The listing builds one solid part. Answer for the finished solid, in the listing's coordinates (mm). Face numbers are marked on the shaded views. A direction names the side the tool comes from. Coordinates: 2 decimals unless noted, no trailing zeros. Loops run counter-clockwise (first coordinate to the right, second up) from the corner with the lowest first, then second, coordinate; pieces in that order, holes last. Notation, with made-up numbers: (23.25, 70) -> (30.25, 70) arc R28 cw to (30.25, 88) -> close; hole circle Ø1 at (0.25, -17). An arc over 180 degrees is marked (long way). Answer in a Markdown table with one row per item.
```python
from build123d import *

# Parameters (mm, degrees)
F0_R       = 22.225
F1_DEPTH   = 76.2
F0_R_2     = 31.75
F2_DEPTH   = 50
F3_SIZE    = 3
F9_D       = 6.8
F9_ON_F7_D = 6.8


with BuildPart() as f1:
    # F0 (on Top) → F1 (new body)
    with BuildSketch(Plane.XY):
        Circle(F0_R)
    extrude(amount=-F1_DEPTH)

    # F0 (on Top) → F2 (join)
    with BuildSketch(Plane.XY):
        Circle(F0_R_2)
        Circle(F0_R, mode=Mode.SUBTRACT)
        Circle(F0_R)
    extrude(amount=F2_DEPTH)

    # F3
    f3_edges = [f1.edges().sort_by_distance(p)[0] for p in [
        (-31.75, 0, 50),
        (-22.225, 0, -76.2),
    ]]
    chamfer(f3_edges, length=F3_SIZE)

    # F9 (through all)
    with Locations(Plane.XZ.offset(31.75)):
        with Locations((0, 25)):
            Hole(F9_D / 2)

    # F9 on F7 (through all)
    with Locations(Plane.YZ.offset(31.75)):
        with Locations((0, 25)):
            Hole(F9_ON_F7_D / 2)


solid = f1.part
```
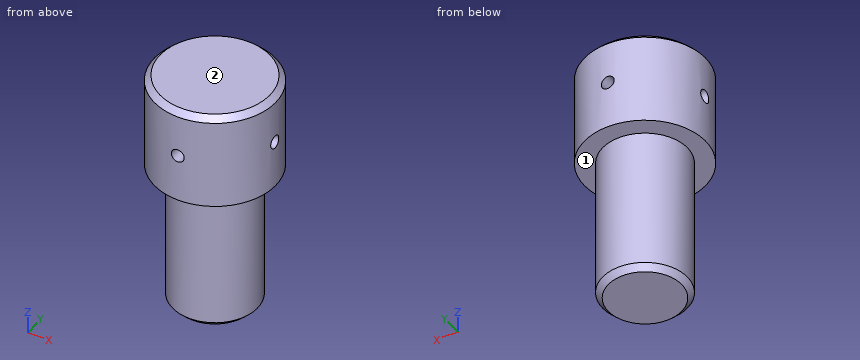
Item 1: A tool of negligible diameter and unlimited length cuts with its end or side. For the marked faces 1 and 2, from which of +Z, -Z, +X, -X, +Y, -Y can it reach the whole face along a straight path? Write none if from no direction.
Findings below:
| item | result |
|---|---|
| face 1 | -Z |
| face 2 | +Z, +X, -X, +Y, -Y |
Item 2: A cutting plane is placed at A-A, the plane z = 25. Determine the outline of the cut face in (x, y).
Findings below:
| item | result |
|---|---|
| outline | (-31.57, -3.4) arc R31.75 ccw to (-3.4, -31.57) -> (-3.4, -3.4) -> close; (-31.57, 3.4) -> (-3.4, 3.4) -> (-3.4, 31.57) arc R31.75 ccw to start; (3.4, -31.57) arc R31.75 ccw to (31.57, -3.4) -> (3.4, -3.4) -> close; (3.4, 3.4) -> (31.57, 3.4) arc R31.75 ccw to (3.4, 31.57) -> close |
Item 3: Find the intervals of material crossed by probe 1 along Z at (x, y) = (-13, 0); probe 2 along Z at (x, y) = (-11, 21); probe 3 along Y at (x, z) = (15.5, 25), in increasing order.
Findings below:
| item | result |
|---|---|
| probe 1 | z = -76.2 to 21.6, 28.4 to 50 |
| probe 2 | z = 0 to 50 |
| probe 3 | y = -27.71 to -3.4, 3.4 to 27.71 |
Item 4: Flat-ended cylindrical pins translate along their axes: pin 1 Ø10 at (x, z) = (8.5, -15) entering from +Y; pin 2 Ø8 at (y, z) = (-9.5, 1) entering from -X; pin 3 Ø6 at (y, z) = (-20, -26) entering from +X. Find the tip coordinate at first contact, or state that the pin passes through.
Findings below:
| item | result |
|---|---|
| pin 1 | stops at y = 21.95 |
| pin 2 | stops at x = -31.27 |
| pin 3 | stops at x = 14.32 |
Item 5: A cutting plane is placed at B-B, the plane z = -50. Determine the outline of the cut face in (x, y) (3 decimals).
Findings below:
| item | result |
|---|---|
| outline | circle Ø44.45 at (0, 0) |
